from build123d import *

# Parameters (mm, degrees)
F0_W     = 127
F0_H     = 285.75
F1_DEPTH = 19.05
F3_DEPTH = 6.35
F4_R     = 3.175
F5_DEPTH = 12.701


with BuildPart() as f1:
    # F0 (on Front) → F1 (new body)
    with BuildSketch(Plane.XZ):
        Rectangle(F0_W, F0_H)
    extrude(amount=F1_DEPTH)

    # F2 (on face) → F3 (cut)
    with BuildSketch(Plane(origin=(0, 0, 0), x_dir=(-1, 0, 0), z_dir=(0, 1, 0))):
        with BuildLine():
            Line((12.7, 104.775), (12.7, 142.875))
            ThreePointArc((12.7, 142.875), (0, 155.575), (-12.7, 142.875))
            Line((-12.7, 142.875), (-12.7, 104.775))
            ThreePointArc((-12.7, 104.775), (0, 92.075), (12.7, 104.775))
        make_face()
    extrude(amount=-F3_DEPTH, mode=Mode.SUBTRACT)

    # F4 (on face) → F5 (cut, through all)
    with BuildSketch(Plane(origin=(0, -6.35, 0), x_dir=(-1, 0, 0), z_dir=(0, 1, 0))):
        with Locations((0, 104.775)):
            Circle(F4_R)
        with Locations((0, 130.175)):
            Circle(F4_R)
    extrude(amount=-F5_DEPTH, mode=Mode.SUBTRACT)


solid = f1.part
CAD build for the part. Positions are in the model's coordinates, mm. A direction names the side the tool comes from. Give positions to 0.01 mm unless a question says otherwise; leave off trailing zeros. Write each loop counter-clockwise with the first axis right and the second up, starting at its lowest first coordinate (ties: lowest second). Pieces come first, ordered by that corner, then holes. Notation, with made-up numbers: (61.5, -31) -> (83.5, -31) arc R29 cw to (83.5, 6) -> close; hole circle Ø1 at (4, 78.5). An arc over 180 degrees is marked (long way). Return JSON: item names as keys, results as strings.
Item 1: Tool access for faces 1 (the flat face through (-1, -19.05, 2)), 2 (the flat face through (0, -6.35, 118)): list every direction of +Z, -Z, +X, -X, +Y, -Y with a clear straight run to the whole face (end or side of a thin tool).
Answer below:
{"face 1": "+Z, -Z, +X, -X, -Y", "face 2": "+Z, +Y"}
Item 2: Band-saw the part on A-A (x = 0). List the corners of the cut face in (y, z) (3 decimals), then the cut area to 3 significant figures.
Answer below:
{"outline": "(-19.05, -142.875) -> (0, -142.875) -> (0, 92.075) -> (-6.35, 92.075) -> (-6.35, 101.6) -> (-19.05, 101.6) -> close; (-19.05, 107.95) -> (-6.35, 107.95) -> (-6.35, 127) -> (-19.05, 127) -> close; (-19.05, 133.35) -> (-6.35, 133.35) -> (-6.35, 142.875) -> (-19.05, 142.875) -> close", "area": "4,960 mm2"}
Item 3: Two-plate mould, pull along Z, no slides. Class faces 3 (the cylindrical face through (0.688, -12.611, 101.676)), 4 (the cylindrical face through (0.413, -12.611, 133.323)), 5 (the flat face through (-1, -9, 142.875)), 6 (the flat face through (-1, 0, 2)): +Z half, -Z half, draft (parallel to the pull), parting line (faces both ways), or undercut.
Answer below:
{"face 3": "undercut", "face 4": "undercut", "face 5": "+Z half", "face 6": "draft"}
Item 4: Drill centre lines: probe 1 along Z at (x, y) = (0, -9.5) (3 decimals); probe 2 along Y at (x, z) = (8, 124); probe 3 along X at (y, z) = (-15.5, 102.5). Where is each one in solid material? Low to high.
Answer below:
{"probe 1": "z = -142.875 to 101.6, 107.95 to 127, 133.35 to 142.875", "probe 2": "y = -19.05 to -6.35", "probe 3": "x = -63.5 to -2.21, 2.21 to 63.5"}
Item 5: Drop flat-ended pins along their axis: pin 1 (6 mm diameter, centred on x = -31.5, z = -94.5, fed in from +Y); pin 2 (7.5 mm diameter, centred on x = 4, z = 124, fed in from +Y). Give the stop position or say it passes through.
Answer below:
{"pin 1": "stops at y = 0", "pin 2": "stops at y = -6.35"}
